Autodesk Inventor part; units mm, degrees
ref_plane "Work Plane1" through (100, 0, 0) normal (1, 0, 0) x (0, 1, 0)
ref_plane "Work Plane2" through (0, 0, -50) normal (0, 0, 1) x (1, 0, 0)
ref_plane "Work Plane3" through (0, 70, 0) normal (0, 1, 0) x (-1, 0, 0)
sketch "Sketch1" plane through (0, 0, 0) normal (0, 0, 1) x (1, 0, 0)
  line L0 (0, 0) -> (100, 0)
  line L1 (100, 0) -> (100, 50)
  line L2 (100, 50) -> (0, 50)
  line L3 (0, 50) -> (0, 0)
  dimension "d0" = 100
  dimension "d1" = 50
sketch "Sketch2" plane through (0, 0, 0) normal (0, 1, 0) x (-1, 0, 0)
  line L0 (0, 0) -> (-100, 0)
  line L1 (-100, 0) -> (-100, -50)
  line L2 (-100, -50) -> (0, -50)
  line L3 (0, -50) -> (0, 0)
  dimension "d2" = 100
  dimension "d3" = 50
sketch "Sketch3" plane through (0, 0, 0) normal (1, 0, 0) x (0, 1, 0)
  line L0 (0, 0) -> (50, 0)
  line L1 (50, 0) -> (50, -50)
  line L2 (50, -50) -> (0, -50)
  line L3 (0, -50) -> (0, 0)
  line L4 (50, -50) -> (70, -50)
  line L5 (70, -50) -> (70, -20)
  line L6 (70, -20) -> (50, -20)
  line L7 (70, -20) -> (50, 0)
  line L8 (70, -20) -> (69, -20)
  line L9 (50, 0) -> (50, -1)
  line L10 (50, -1) -> (69, -20)
  dimension "d16" = 50
  dimension "d17" = 50
  dimension "d18" = 20
  dimension "d19" = 30
  dimension "d20" = 1
extrude "Extrusion1" add sketch "Sketch1" against normal blind 1
extrude "Extrusion2" add sketch "Sketch2" along normal blind 1
extrude "Extrusion3" add sketch "Sketch3" along normal blind 1
ref_plane "Work Plane1" through (100, 0, 0) normal (1, 0, 0) x (0, 1, 0)
sketch "Sketch4" plane through (100, 0, 0) normal (1, 0, 0) x (0, 1, 0)
  line L0 (0, 0) -> (0, -50)
  line L1 (70, -50) -> (70, -20)
  line L2 (0, -50) -> (70, -50)
  line L3 (70, -50) -> (70, -20)
  line L4 (50, 0) -> (50, -1)
  line L5 (50, 0) -> (50, -1)
  line L6 (50, -1) -> (69, -20)
  line L7 (69, -20) -> (70, -20)
  line L8 (0, -50) -> (50, -50)
  line L9 (1, -50) -> (70, -50)
  line L10 (50, -1) -> (50, -50)
  line L11 (0, 0) -> (50, 0)
  line L12 (0, 0) -> (50, 0)
  point P0 (-1, 0)
extrude "Extrusion4" add sketch "Sketch4" along normal blind 1
ref_plane "Work Plane2" through (0, 0, -50) normal (0, 0, 1) x (1, 0, 0)
sketch "Sketch5" plane through (0, 0, -50) normal (0, 0, 1) x (1, 0, 0)
  line L0 (101, 0) -> (101, 70)
  line L1 (0, 0) -> (101, 0)
  line L2 (101, 0) -> (101, 70)
  line L3 (101, 70) -> (0, 70)
  line L4 (0, 70) -> (0, 0)
  dimension "d27" = 101
  dimension "d28" = 70
sketch "Sketch6" plane through (101, 0, 0) normal (1, 0, 0) x (0, 0, -1)
  line L0 (1, 50) -> (0, 50)
  line L1 (20, 69) -> (1, 50)
  line L2 (0, 50) -> (1, 50)
  line L3 (1, 50) -> (20, 69)
  line L4 (20, 70) -> (20, 69)
  line L5 (20, 69) -> (20, 70)
  line L6 (20, 70) -> (0, 50)
  point P0 (0, 0)
extrude "Extrusion5" add sketch "Sketch6" against normal blind 100
extrude "Extrusion6" add sketch "Sketch5" along normal blind 1
ref_plane "Work Plane3" through (0, 70, 0) normal (0, 1, 0) x (-1, 0, 0)
sketch "Sketch7" plane through (0, 70, 0) normal (0, 1, 0) x (-1, 0, 0)
  line L0 (0, -50) -> (-101, -50)
  line L1 (-101, -50) -> (-101, -20)
  line L2 (0, -50) -> (-101, -50)
  line L3 (-101, -50) -> (-101, -20)
  line L4 (-101, -20) -> (0, -20)
  line L5 (0, -20) -> (0, -50)
  point P0 (0, 0)
extrude "Extrusion7" add sketch "Sketch7" against normal blind 1
properties part number "Design inkubator"
Can you work these out from the model? Positions are in its coordinate system, mm. A direction names the side the tool comes from. Give positions to 0.01 mm unless a question says otherwise; leave off trailing zeros. Write each loop counter-clockwise with the first axis right and the second up, starting at its lowest first coordinate (ties: lowest second). Pieces come first, ordered by that corner, then holes. Notation, with made-up numbers: (77, 43) -> (118, 43) arc R22 ccw to (118, 61) -> close; hole circle Ø11 at (72.25, 78.25). An arc over 180 degrees is marked (long way). Write item = value, one per line.
(1) Suppose I cut it at C-C on z = -15. Write out the boundary of the cut face in (x, y), then the cut area to 3 significant figures.
Worked out:
outline = (0, 0) -> (101, 0) -> (101, 65) -> (0, 65) -> close; hole (1, 1) -> (100, 1) -> (100, 64) -> (1, 64) -> close
area = 328 mm^2
(2) I need wall thicknesses on probe 1 along X at (y, z) = (63.5, -30.5); probe 2 along Y at (x, z) = (57, -43.5); probe 3 along Z at (x, y) = (95, 26). Which ranges of each line are inside material? Lowest first, please. Write a range as from..to.
Worked out:
probe_1 = 0..1, 100..101
probe_2 = 0..1, 69..70
probe_3 = -50..-49, -1..0
(3) For faces 1 (the face through (50, 26, -1)), 2 (the face through (0, 35, -25)), which set-ups out of +Z, -Z, +X, -X, +Y, -Y let a thin tool reach every point of the face, with its end or its side?
Worked out:
face_1 = none
face_2 = +Z, -Z, -X, +Y, -Y
(4) Suppose I cut it at A-A on x = 55. Write out the boundary of the cut face in (y, z).
Worked out:
outline = (0, -50) -> (70, -50) -> (70, -20) -> (50, 0) -> (0, 0) -> close; hole (1, -49) -> (69, -49) -> (69, -20) -> (50, -1) -> (1, -1) -> close
(5) Suppose I cut it at B-B on y = 8.5. Write out the boundary of the cut face in (x, z).
Worked out:
outline = (0, -50) -> (101, -50) -> (101, 0) -> (0, 0) -> close; hole (1, -49) -> (100, -49) -> (100, -1) -> (1, -1) -> close
(6) Thinking about a two-plate mould opening in Y: for faces 3 (the face through (51, 60, -10)), 4 (the face through (50, 35, -49)), 5 (the face through (50, 25, 0)), which applies, released by +Y, released by -Y, zero draft, split by the parting line, or undercut?
Worked out:
face_3 = released by +Y
face_4 = undercut
face_5 = zero draft
